from build123d import *

# Parameters (mm, degrees)
F0_W      = 52.3875
F0_H      = 44.45
F1_DEPTH  = 3.175
F3_DEPTH  = 3.176
F4_R      = 3.5687
F5_DEPTH  = 9.525
F6_R      = 2.778125
F7_DEPTH  = 12.701
F9_DEPTH  = 9.525
F10_R     = 3.175
F11_DEPTH = 3.176


with BuildPart() as f1:
    # F0 (on Front) → F1 (new body)
    with BuildSketch(Plane.XZ):
        with Locations((1.981661, -2.357554)):
            Rectangle(F0_W, F0_H)
    extrude(amount=F1_DEPTH)

    # F2 (on face) → F3 (cut, through all)
    with BuildSketch(Plane.XZ.offset(3.175)):
        with BuildLine():
            ThreePointArc((-14.290214, 13.517446), (-17.862089, 17.089321), (-21.433964, 13.517446))
            ThreePointArc((-21.433964, 13.517446), (-17.862089, 9.945571), (-14.290214, 13.517446))
        make_face()
    extrude(amount=-F3_DEPTH, mode=Mode.SUBTRACT)

    # F4 (on face) → F5 (join)
    with BuildSketch(Plane.XZ.offset(3.175)):
        with Locations((21.825411, 13.517446)):
            Circle(F4_R)
    extrude(amount=F5_DEPTH)

    # F6 (on face) → F7 (cut, through all)
    with BuildSketch(Plane.XZ.offset(12.7)):
        with Locations((21.825411, 13.517446)):
            Circle(F6_R)
    extrude(amount=-F7_DEPTH, mode=Mode.SUBTRACT)

    # F8 (on face) → F9 (join)
    with BuildSketch(Plane.XZ.offset(3.175)):
        with BuildLine():
            ThreePointArc((-14.687089, -18.232554), (-17.862089, -15.057554), (-21.037089, -18.232554))
            ThreePointArc((-21.037089, -18.232554), (-17.862089, -21.407554), (-14.687089, -18.232554))
        make_face()
    extrude(amount=F9_DEPTH)

    # F10 (on face) → F11 (cut, through all)
    with BuildSketch(Plane.XZ.offset(3.175)):
        with Locations((21.825411, -18.232554)):
            Circle(F10_R)
    extrude(amount=-F11_DEPTH, mode=Mode.SUBTRACT)


solid = f1.part
Could you check a few things on this model? Use its own coordinates, in mm. A direction names the side the tool comes from. Coordinates: 2 decimals unless noted, no trailing zeros. Order: outer loops, then holes, each group sorted by start corner. A loop starts at its lowest first (then second) coordinate and runs counter-clockwise, first axis right, second up.
Q1. Suppose I cut it at C-C on z = 12. Please give me the cut outline in (x, y) (1 decimal).
Q2. Suppose I cut it at A-A on z = -17. Please give me the cut outline in (x, y) (3 decimals), and give its area (3 significant figures).
Q3. Suppose I cut it at B-B on x = -20. Please give me the cut outline in (y, z) (3 decimals).
Q4. Which directions (+Z, -Z, +X, -X, +Y, -Y) give clear straight access to the entire face, cutting with the end or side of a thin tool? Please do faces 4 (the cylindrical face through (25.12, -7.87, 12.15)), 5 (the flat face through (2, 0, -2)).
Q5. Thinking about a two-plate mould opening in X: for faces 1 (the flat face through (24, -12.7, 11)), 2 (the flat face through (-24.212, -2, -3)), 3 (the cylindrical face through (-21.269, -1.61, 12.445)), which applies, released by +X, released by -X, zero draft, split by the parting line, or undercut?
Q6. Suppose I cut it at D-D on y = -2.5. Please give me the cut outline in (x, z) (3 decimals), and give its area (3 significant figures).
Q7. Will these pins go through, and if not, where does the flat tip stop? pin 1 (22 mm diameter, centred on x = -5, z = -2, fed in from -Y) (3 decimals); pin 2 (1 mm diameter, centred on y = -7.5, z = 12, fed in from +X).
Q8. Please list where these lines run through material, in increasing order: L1, parallel to Y at x = 20, z = 7 (3 decimals); L2, parallel to Z at x = -16.5, y = -1.5; L3, parallel to X at y = -10.25, z = 11.
Answer:
1. outline: (-24.2, -3.2) - (-21.1, -3.2) - (-21.1, 0) - (-24.2, 0) - close; (-14.6, -3.2) - (18.6, -3.2) - (18.6, -12.7) - (19.5, -12.7) - (19.5, 0) - (-14.6, 0) - close; (24.2, -12.7) - (25.1, -12.7) - (25.1, -3.2) - (28.2, -3.2) - (28.2, 0) - (24.2, 0) - close
2. outline: (-24.212, -3.175) - (-20.788, -3.175) - (-20.788, -12.7) - (-14.936, -12.7) - (-14.936, -3.175) - (18.899, -3.175) - (18.899, 0) - (-24.212, 0) - close; (24.751, -3.175) - (28.175, -3.175) - (28.175, 0) - (24.751, 0) - close
2. area: 203 mm2
3. outline: (-12.7, -20.58) - (-3.175, -20.58) - (-3.175, -24.583) - (0, -24.583) - (0, 10.656) - (-3.175, 10.656) - (-3.175, -15.885) - (-12.7, -15.885) - close; (-3.175, 16.379) - (0, 16.379) - (0, 19.867) - (-3.175, 19.867) - close
4. face 4: -Y
4. face 5: +Z, -Z, +X, -X, +Y
5. face 1: zero draft
5. face 2: released by -X
5. face 3: undercut
6. outline: (-24.212, -24.583) - (28.175, -24.583) - (28.175, 19.867) - (-24.212, 19.867) - close; hole circle Ø7.144 at (-17.862, 13.517); hole circle Ø6.35 at (21.825, -18.233); hole circle Ø5.556 at (21.825, 13.517)
6. area: 2,230 mm2
7. pin 1: stops at y = -3.175
7. pin 2: stops at x = 25.25
8. L1: y = -3.175 to 0
8. L2: z = -24.58 to 10.22, 16.82 to 19.87
8. L3: x = 19.3 to 20.65, 23 to 24.35
